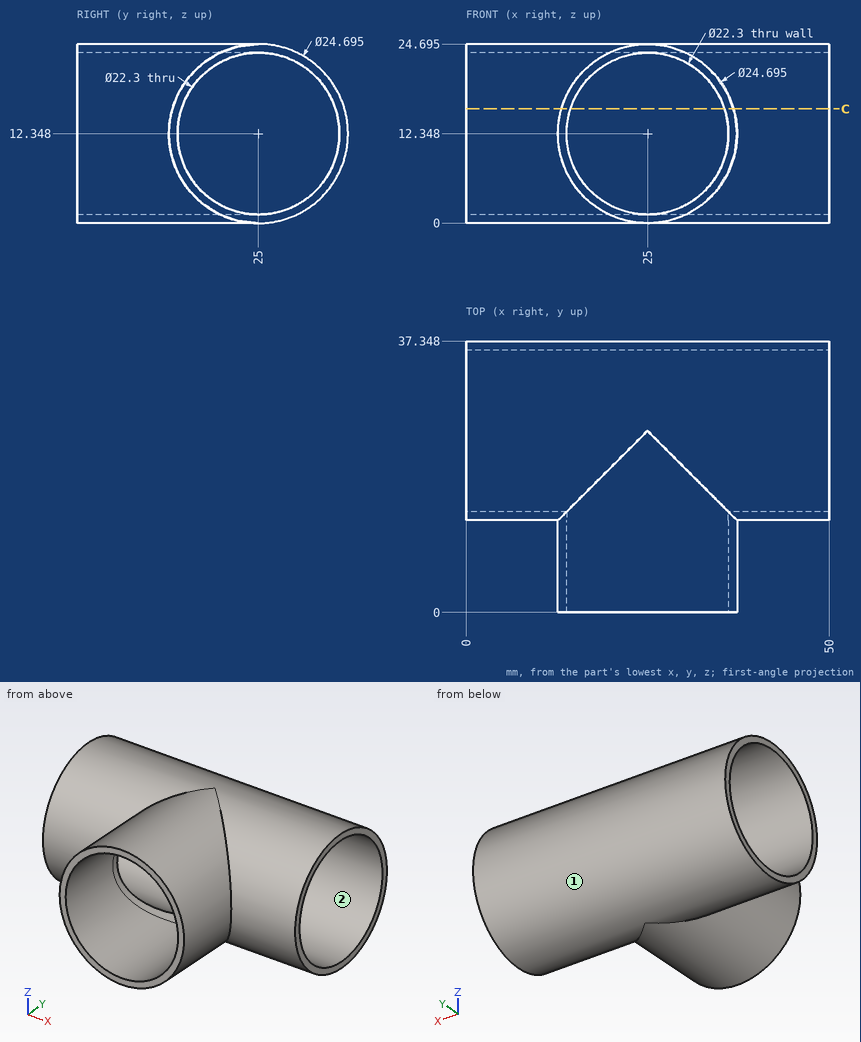
Geometry: see drawing. Coordinates: mm, zero at the bounding-box minimum. Give positions to 0.01 mm unless a question says otherwise; leave off trailing zeros. Loops run counter-clockwise (first coordinate to the right, second up) from the corner with the lowest first, then second, coordinate; pieces in that order, holes last. Notation, with made-up numbers: (-34.75, 46) -> (13.25, 46) arc R9 cw to (13.25, 60) -> close; hole circle Ø9 at (-21, -37.75). An arc over 180 degrees is marked (long way). Answer as a JSON object with one key per item and string values. Group by question number.
Item 1: Pin query (flat end, axial travel): P1, Ø5, axis at x = 19.5, z = 12, coming from the -Y side; P2, Ø4, axis at x = 28, y = 28, coming from the +Z side (1 decimal); P3, Ø2, axis at x = 6, z = 3.5, coming from the -Y side. Return the tip coordinate at first contact, or that it passes through.
Item 2: Cut plane C-C, the plane z = 15.75. Return the cut outline in (x, y).
Item 3: Pull-direction query (Y, two-part tool) for the marked faces 1 and 2; classes: released by +Y, released by -Y, zero draft, split by the parting line, or undercut.
Item 4: Line query: probe 1 along Z at (x, y) = (25, 19) (1 decimal); probe 2 along Y at (x, z) = (8, 12.5); probe 3 along Y at (x, z) = (8.5, 6.75) (1 decimal). Output: solid intervals per line, ascending.
Checks:
{
 "1": {"P1": "stops at y = 35.78", "P2": "stops at z = 24.7", "P3": "stops at y = 15.47"},
 "2": {"outline": "(0, 13.13) -> (13.13, 13.13) -> (13.13, 0) -> (14.38, 0) -> (14.38, 14.38) -> (0, 14.38) -> close; (0, 35.62) -> (50, 35.62) -> (50, 36.87) -> (0, 36.87) -> close; (35.62, 0) -> (36.87, 0) -> (36.87, 13.13) -> (50, 13.13) -> (50, 14.38) -> (35.62, 14.38) -> close"},
 "3": {"face 1": "split by the parting line", "face 2": "undercut"},
 "4": {"probe 1": "z = 0 to 1.2, 23.5 to 24.7", "probe 2": "y = 12.65 to 13.85, 36.15 to 37.35", "probe 3": "y = 14 to 15.4, 34.6 to 36"}
}
